Input: part model. Units: mm. Frame: model coordinates. A direction names the side the tool comes from. Give positions to 0.01 mm unless a question says otherwise; leave off trailing zeros. Write each loop counter-clockwise with the first axis right and the second up, starting at its lowest first coordinate (ties: lowest second). Pieces come first, ordered by that corner, then holes. Notation, with made-up numbers: (61, 66) - (81, 66) arc R13 ccw to (81, 84) - close; hole circle Ø3 at (77.25, -18). An arc over 180 degrees is marked (long way). Answer as a JSON object with one key per item and string values. Group by question number.
from build123d import *

# Parameters (mm, degrees)
SKETCH_1_R          = 6
SKETCH_1_R_2        = 5
EXTRUDE_1_DEPTH     = 14
CUT_EXTRUDE_1_DEPTH = 1
CUT_EXTRUDE_START   = -1
CUT_EXTRUDE_2_DEPTH = 1


with BuildPart() as part:
    # 草图1 → 拉伸1 (new body)
    with BuildSketch(Plane.XY):
        with BuildLine():
            Line((-8, 121.801117832), (-13.5, 18.135932445))
            ThreePointArc((-13.5, 18.135932445), (-14.135015735, 15.121742333), (-15.657303504, 12.443827667))
            ThreePointArc((-15.657303504, 12.443827667), (0, -20), (15.657303504, 12.443827667))
            ThreePointArc((15.657303504, 12.443827667), (14.135015735, 15.121742333), (13.5, 18.135932445))
            Line((13.5, 18.135932445), (8, 121.801117832))
            ThreePointArc((8, 121.801117832), (8.376311259, 125.097647375), (9.810521048, 128.089596484))
            ThreePointArc((9.810521048, 128.089596484), (0, 147), (-9.810521048, 128.089596484))
            ThreePointArc((-9.810521048, 128.089596484), (-8.376311259, 125.097647375), (-8, 121.801117832))
        make_face()
        Circle(SKETCH_1_R, mode=Mode.SUBTRACT)
        with Locations((0, 135)):
            Circle(SKETCH_1_R_2, mode=Mode.SUBTRACT)
    extrude(amount=-EXTRUDE_1_DEPTH)

    # 草图2 → 切除-拉伸1 (cut)
    with BuildSketch(Plane.XY):
        with BuildLine():
            Line((-3.75192728, 105), (-3.75192728, 55))
            ThreePointArc((-3.75192728, 55), (0.24807272, 51), (4.24807272, 55))
            Line((4.24807272, 55), (4.24807272, 105))
            ThreePointArc((4.24807272, 105), (0.24807272, 109), (-3.75192728, 105))
        make_face()
    extrude(amount=-CUT_EXTRUDE_1_DEPTH, mode=Mode.SUBTRACT)

    # 草图3 → 切除-拉伸2 (cut)
    with BuildSketch(Plane(origin=(0, 0, -14), x_dir=(-1, 0, 0), z_dir=(0, 0, -1)).offset(CUT_EXTRUDE_START)):
        with BuildLine():
            Line((3.75192728, 55), (3.75192728, 105))
            ThreePointArc((3.75192728, 105), (-0.24807272, 109), (-4.24807272, 105))
            Line((-4.24807272, 105), (-4.24807272, 55))
            ThreePointArc((-4.24807272, 55), (-0.24807272, 51), (3.75192728, 55))
        make_face()
    extrude(amount=CUT_EXTRUDE_2_DEPTH, mode=Mode.SUBTRACT)


solid = part.part
1) Cut plane B-B on z = -8. Return the cut outline in (x, y), and give its area (3 significant figures).
2) Pin query (flat end, axial travel): P1, Ø5, axis at x = 9, z = -10.5, coming from the -Y side; P2, Ø1, axis at y = 83, z = -7.5, coming from the -X side; P3, Ø0.8, axis at y = 67.5, z = -13.5, coming from the +X side. Return the tip coordinate at first contact, or that it passes through.
3) Cut plane A-A on y = 135. Return the cut outline in (x, z), and give its area (3 significant figures).
4) Mould query, pull axis X, two halves, no side actions, for faces 4 (the face through (10.79, 69.24, -6.9)), 5 (the face through (0, 80, -13)), 6 (the face through (0, 46, -14)). Classes: +X half, -X half, draft (parallel to the pull), parting line (faces both ways), or undercut.
5) Reachability of faces 1 (the face through (0.3, 109, -0.5)), 2 (the face through (0.3, 51, -13.5)), 3 (the face through (-8.39, 125.14, -6.9)) from +Z, -Z, +X, -X, +Y, -Y: full face, straight path, thin tool, end or side. Return the list, or none.
6) Cut plane D-D on y = 0. Return the cut outline in (x, z), and give its area (3 significant figures).
7) Line query: line 1 along Y through (x, z) = (0, -6.75); line 2 along Z through (x, y) = (-2, 56); line 3 along Y through (x, z) = (4, -9.75). Output: solid intervals per line, ascending. Write a range as from..to.
8) Cut plane C-C on x = 2. Return the cut outline in (y, z).
Filled in:
{
 "1": {"outline": "(-15.66, 12.44) arc R20 ccw (long way) to (15.66, 12.44) arc R10 cw to (13.5, 18.14) - (8, 121.8) arc R10 cw to (9.81, 128.09) arc R12 ccw (long way) to (-9.81, 128.09) arc R10 cw to (-8, 121.8) - (-13.5, 18.14) arc R10 cw to start; hole circle Ø12 at (0, 0); hole circle Ø10 at (0, 135)", "area": "3,780 mm²"},
 "2": {"P1": "stops at y = -18.91", "P2": "stops at x = -10.09", "P3": "stops at x = 10.9"},
 "3": {"outline": "(-12, -14) - (-5, -14) - (-5, 0) - (-12, 0) - close; (5, -14) - (12, -14) - (12, 0) - (5, 0) - close", "area": "196 mm²"},
 "4": {"face 4": "+X half", "face 5": "undercut", "face 6": "draft"},
 "5": {"face 1": "+Z", "face 2": "-Z", "face 3": "+Z, -Z, -X"},
 "6": {"outline": "(-20, -14) - (-6, -14) - (-6, 0) - (-20, 0) - close; (6, -14) - (20, -14) - (20, 0) - (6, 0) - close", "area": "392 mm²"},
 "7": {"line 1": "y = -20..-6, 6..130, 140..147", "line 2": "z = -13..-1", "line 3": "y = -19.6..-4.47, 4.47..132, 138..146.31"},
 "8": {"outline": "(-19.9, -14) - (-5.66, -14) - (-5.66, 0) - (-19.9, 0) - close; (5.66, -14) - (51.4, -14) - (51.4, -13) - (108.6, -13) - (108.6, -14) - (130.42, -14) - (130.42, 0) - (108.6, 0) - (108.6, -1) - (51.4, -1) - (51.4, 0) - (5.66, 0) - close; (139.58, -14) - (146.83, -14) - (146.83, 0) - (139.58, 0) - close"}
}
